Build history of the part. All positions in model axes, mm. Give positions to 0.01 mm unless a question says otherwise; leave off trailing zeros. Order: outer loops, then holes, each group sorted by start corner. A loop starts at its lowest first (then second) coordinate and runs counter-clockwise, first axis right, second up. Notation, with made-up numbers: (-37, 65.5) -> (-20, 65.5) arc R12 ccw to (-20, 81.5) -> close; hole circle Ø7 at (-20, 67.5). An arc over 180 degrees is marked (long way). One line per item, written item: value. Start each with the question number.
(1) Saw through at D-D on y = -18.5. Give the cut face in (x, z).
(2) Saw through at A-A on y = 0. Give the cut face in (x, z).
(3) Two-plate mould, pull along Y, no slides. Class faces 1 (the cylindrical face through (6.261, -11.444, 23.555)), 2 (the cylindrical face through (6.26, 10.6, 3.34)), 3 (the flat face through (0, 5, -11)): +Y half, -Y half, draft (parallel to the pull), parting line (faces both ways), or undercut.
(4) Saw through at C-C on z = -9. Give the cut face in (x, y).
(5) Pin check, flat tips, straight feed: pin 1 (5 mm diameter, centred on x = 5.5, y = 18, fed in from +Z); pin 2 (5 mm diameter, centred on x = 8.5, z = 1, fed in from +Y). Stop position of each tip, or through.
(6) Probe line 1 (Z direction, x = 7.25, y = 0); line 2 (Y direction, x = 11.5, z = -10); line 3 (Z direction, x = 11.75, y = -7). List the from-to ranges inside material, lowest first.
(7) Saw through at B-B on x = 1. Give the cut face in (y, z) (1 decimal), plus the area to 3 significant figures.
```python
from build123d import *

# Parameters (mm, degrees)
F0_R     = 11.1125
F1_DEPTH = 12.7


with BuildPart() as f1:
    # F0 (on Right) → F1 (new body)
    with BuildSketch(Plane.YZ):
        with BuildLine():
            Line((4.850968, 25.4), (0, 25.4))
            Line((0, 25.4), (-4.850968, 25.4))
            ThreePointArc((-4.850968, 25.4), (-11.527753, 23.503265), (-16.210194, 18.379613))
            Line((-16.210194, 18.379613), (-24.059225, 2.681549))
            ThreePointArc((-24.059225, 2.681549), (-25.060262, -0.080201), (-25.4, -2.998063))
            Line((-25.4, -2.998063), (-25.4, -25.4))
            Line((-25.4, -25.4), (0, -25.4))
            Line((0, -25.4), (25.4, -25.4))
            Line((25.4, -25.4), (25.4, -2.998063))
            ThreePointArc((25.4, -2.998063), (25.060262, -0.080201), (24.059225, 2.681549))
            Line((24.059225, 2.681549), (16.210194, 18.379613))
            ThreePointArc((16.210194, 18.379613), (11.527753, 23.503265), (4.850968, 25.4))
        make_face()
        Circle(F0_R, mode=Mode.SUBTRACT)
    extrude(amount=F1_DEPTH)


solid = f1.part
```
Results below:
1. outline: (0, -25.4) -> (12.7, -25.4) -> (12.7, 13.8) -> (0, 13.8) -> close
2. outline: (0, -25.4) -> (12.7, -25.4) -> (12.7, -11.11) -> (0, -11.11) -> close; (0, 11.11) -> (12.7, 11.11) -> (12.7, 25.4) -> (0, 25.4) -> close
3. face 1: -Y half
3. face 2: undercut
3. face 3: draft
4. outline: (0, -25.4) -> (12.7, -25.4) -> (12.7, -6.52) -> (0, -6.52) -> close; (0, 6.52) -> (12.7, 6.52) -> (12.7, 25.4) -> (0, 25.4) -> close
5. pin 1: stops at z = 19.62
5. pin 2: stops at y = 25.31
6. line 1: z = -25.4 to -11.11, 11.11 to 25.4
6. line 2: y = -25.4 to -4.85, 4.85 to 25.4
6. line 3: z = -25.4 to -8.63, 8.63 to 25.22
7. outline: (-25.4, -25.4) -> (25.4, -25.4) -> (25.4, -3) arc R12.7 ccw to (24.1, 2.7) -> (16.2, 18.4) arc R12.7 ccw to (4.9, 25.4) -> (-4.9, 25.4) arc R12.7 ccw to (-16.2, 18.4) -> (-24.1, 2.7) arc R12.7 ccw to (-25.4, -3) -> close; hole circle Ø22.2 at (0, 0)
7. area: 1,850 mm²
